from build123d import *

# Parameters (mm, degrees)
F0_W      = 60
F0_H      = 80
F2_DEPTH  = 46
F1_W      = 30
F1_H      = 10
F3_DEPTH  = 10
F4_W      = 44
F4_H      = 64
F5_DEPTH  = 30
F6_W      = 8
F6_H      = 48
F7_DEPTH  = 30
F8_W      = 22
F8_H      = 30
F8_W_2    = 8
F9_DEPTH  = 8
F10_R     = 20
F12_DEPTH = 8
F14_DEPTH = 40
F15_R     = 5
F17_DEPTH = 8
F18_R     = 5
F19_W     = 7
F19_H     = 8
F20_DEPTH = 5
F21_W     = 22
F21_H     = 30
F21_W_2   = 8
F22_DEPTH = 8
F23_SIZE2 = 29.99999
F23_SIZE  = 21.99999
F25_DEPTH = 8
F27_DEPTH = 40
F29_DEPTH = 8


# Not quite as in the source:
# - a fillet or chamfer is up to 0.001 mm smaller than in the source, because OpenCascade refuses the exact size


with BuildPart() as f2:
    # F0 (on Top) → F2 (new body)
    with BuildSketch(Plane.XY):
        Rectangle(F0_W, F0_H)
    extrude(amount=F2_DEPTH)

    # F1 (on face) → F3 (cut)
    with BuildSketch(Plane.XY):
        with Locations((-15, 30)):
            Rectangle(F1_W, F1_H)
        with Locations((15, -30)):
            Rectangle(F1_W, F1_H)
    extrude(amount=F3_DEPTH, mode=Mode.SUBTRACT)

    # F4 (on face) → F5 (cut)
    with BuildSketch(Plane.XY.offset(46)):
        Rectangle(F4_W, F4_H)
    extrude(amount=-F5_DEPTH, mode=Mode.SUBTRACT)

    # F6 (on face) → F7 (cut, through all)
    with BuildSketch(Plane.XY.offset(46)):
        with Locations((-26, 0)):
            Rectangle(F6_W, F6_H)
        with Locations((26, 0)):
            Rectangle(F6_W, F6_H)
    extrude(amount=-F7_DEPTH, mode=Mode.SUBTRACT)

    # F8 (on face) → F9 (join)
    with BuildSketch(Plane(origin=(0, -24, 0), x_dir=(-1, 0, 0), z_dir=(0, 1, 0))):
        with Locations((-41, 31)):
            Rectangle(F8_W, F8_H)
        with Locations((-26, 31)):
            Rectangle(F8_W_2, F8_H)
    extrude(amount=F9_DEPTH)

    # F10
    f10_edges = [f2.edges().sort_by_distance(p)[0] for p in [
        (52, -20, 16),
    ]]
    fillet(f10_edges, radius=F10_R)

    # F11 (on face) → F12 (join, through all)
    with BuildSketch(Plane(origin=(0, -16, 0), x_dir=(-1, 0, 0), z_dir=(0, 1, 0))):
        with BuildLine():
            ThreePointArc((-58.1533936612, 46), (-59.5344785906, 41.08453427), (-60, 36))
            ThreePointArc((-60, 36), (-51.7989898732, 16.2010101268), (-32, 8))
            Line((-32, 8), (-32, 16))
            ThreePointArc((-32, 16), (-46.1421356237, 21.8578643763), (-52, 36))
            Line((-52, 36), (-52, 46))
            Line((-52, 46), (-58.1533936612, 46))
        make_face()
        with BuildLine():
            Line((-60, 46), (-60, 36))
            ThreePointArc((-60, 36), (-59.5344785906, 41.08453427), (-58.1533936612, 46))
            Line((-58.1533936612, 46), (-60, 46))
        make_face()
        with BuildLine():
            Line((-32, 16), (-32, 8))
            ThreePointArc((-32, 8), (-30.999360817, 8.0178856906), (-30, 8.0715199125))
            Line((-30, 8.0715199125), (-30, 16))
            Line((-30, 16), (-32, 16))
        make_face()
    extrude(amount=-F12_DEPTH)

    # F13 (on face) → F14 (join, through all)
    with BuildSketch(Plane(origin=(0, -16, 0), x_dir=(-1, 0, 0), z_dir=(0, 1, 0))):
        with BuildLine():
            ThreePointArc((-58.1533936612, 46), (-59.5344785906, 41.08453427), (-60, 36))
            Line((-60, 36), (-52, 36))
            Line((-52, 36), (-52, 46))
            Line((-52, 46), (-58.1533936612, 46))
        make_face()
        with BuildLine():
            Line((-60, 46), (-60, 36))
            ThreePointArc((-60, 36), (-59.5344785906, 41.08453427), (-58.1533936612, 46))
            Line((-58.1533936612, 46), (-60, 46))
        make_face()
        with BuildLine():
            Line((-52, 36), (-60, 36))
            ThreePointArc((-60, 36), (-51.7989898732, 16.2010101268), (-32, 8))
            Line((-32, 8), (-32, 16))
            ThreePointArc((-32, 16), (-46.1421356237, 21.8578643763), (-52, 36))
        make_face()
        with BuildLine():
            Line((-32, 16), (-32, 8))
            ThreePointArc((-32, 8), (-30.999360817, 8.0178856906), (-30, 8.0715199125))
            Line((-30, 8.0715199125), (-30, 16))
            Line((-30, 16), (-32, 16))
        make_face()
    extrude(amount=F14_DEPTH)

    # F15
    f15_edges = [f2.edges().sort_by_distance(p)[0] for p in [
        (51.078784, -24, 15.506098),
    ]]
    fillet(f15_edges, radius=F15_R)

    # F16 (on face) → F17 (join)
    with BuildSketch(Plane(origin=(0, 24, 0), x_dir=(-1, 0, 0), z_dir=(0, 1, 0))):
        with BuildLine():
            ThreePointArc((-30, 8.0715199125), (-30.999360817, 8.0178856906), (-32, 8))
            Line((-32, 8), (-30, 8))
            Line((-30, 8), (-30, 8.0715199125))
        make_face()
        with BuildLine():
            Line((-30, 16), (-32, 16))
            Line((-32, 16), (-32, 8))
            ThreePointArc((-32, 8), (-30.999360817, 8.0178856906), (-30, 8.0715199125))
            Line((-30, 8.0715199125), (-30, 16))
        make_face()
        with BuildLine():
            ThreePointArc((-32, 16), (-46.1421356237, 21.8578643763), (-52, 36))
            Line((-52, 36), (-60, 36))
            ThreePointArc((-60, 36), (-51.7989898732, 16.2010101268), (-32, 8))
            Line((-32, 8), (-32, 16))
        make_face()
        with BuildLine():
            Line((-60, 46), (-60, 36))
            ThreePointArc((-60, 36), (-59.5344785906, 41.08453427), (-58.1533936612, 46))
            Line((-58.1533936612, 46), (-60, 46))
        make_face()
        with BuildLine():
            Line((-60, 36), (-52, 36))
            Line((-52, 36), (-52, 46))
            Line((-52, 46), (-58.1533936612, 46))
            ThreePointArc((-58.1533936612, 46), (-59.5344785906, 41.08453427), (-60, 36))
        make_face()
        with BuildLine():
            ThreePointArc((-30, 16.1002512579), (-30.9987444988, 16.0250785378), (-32, 16))
            Line((-32, 16), (-30, 16))
            Line((-30, 16), (-30, 16.1002512579))
        make_face()
        with BuildLine():
            ThreePointArc((-49.3205080757, 46), (-51.3185165258, 41.1763809021), (-52, 36))
            ThreePointArc((-52, 36), (-46.1421356237, 21.8578643763), (-32, 16))
            ThreePointArc((-32, 16), (-30.9987444988, 16.0250785378), (-30, 16.1002512579))
            Line((-30, 16.1002512579), (-30, 46))
            Line((-30, 46), (-49.3205080757, 46))
        make_face()
        with BuildLine():
            Line((-52, 46), (-52, 36))
            ThreePointArc((-52, 36), (-51.3185165258, 41.1763809021), (-49.3205080757, 46))
            Line((-49.3205080757, 46), (-52, 46))
        make_face()
    extrude(amount=F17_DEPTH)

    # F18
    f18_edges = [f2.edges().sort_by_distance(p)[0] for p in [
        (51.79899, 32, 16.20101),
    ]]
    fillet(f18_edges, radius=F18_R)

    # F19 (on face) → F20 (join)
    with BuildSketch(Plane.XY.offset(46)):
        with Locations((33.5, 28)):
            Rectangle(F19_W, F19_H)
        with Locations((33.5, -20)):
            Rectangle(F19_W, F19_H)
    extrude(amount=F20_DEPTH)

    # F21 (on face) → F22 (join)
    with BuildSketch(Plane.XZ.offset(-24)):
        with Locations((-41, 31)):
            Rectangle(F21_W, F21_H)
        with Locations((-26, 31)):
            Rectangle(F21_W_2, F21_H)
    extrude(amount=F22_DEPTH)

    # F23 (size 22 and 30 in the source; OpenCascade refuses exactly that, so slightly less here)
    f23_edges = [f2.edges().sort_by_distance(p)[0] for p in [
        (-52, 20, 16),
    ]]
    f23_side = f2.faces().sort_by_distance((-41, 20, 16))[0]
    chamfer(f23_edges, length=F23_SIZE, length2=F23_SIZE2, reference=f23_side)

    # F24 (on face) → F25 (join)
    with BuildSketch(Plane.XZ.offset(-16)):
        Polygon((-30, 16), (-52, 46), (-61.9205734601, 46), (-30, 2.4719452816), align=None)
    extrude(amount=-F25_DEPTH)

    # F26 (on face) → F27 (join, through all)
    with BuildSketch(Plane.XZ.offset(-16)):
        Polygon((-61.9205734601, 46), (-30, 2.4719452816), (-30, 16), (-52, 46), align=None)
    extrude(amount=F27_DEPTH)

    # F28 (on face) → F29 (join)
    with BuildSketch(Plane.XZ.offset(24)):
        Polygon((-51.9714293201, 45.961039982), (-30, 16), (-30, 45.8750016987), align=None)
        Polygon((-61.9205734601, 46), (-30, 2.4719452816), (-30, 16), (-51.9714293201, 45.961039982), align=None)
    extrude(amount=F29_DEPTH)


solid = f2.part
Could you check a few things on this model? Use its own coordinates, in mm. A direction names the side the tool comes from. Round coordinates to 2 decimals unless told otherwise and drop trailing zeros. Write each loop counter-clockwise with the first axis right and the second up, starting at its lowest first coordinate (ties: lowest second). Pieces come first, ordered by that corner, then holes. Notation, with made-up numbers: (9, 16) - (35, 16) arc R25 cw to (35, 44) - close; hole circle Ø10 at (-19, 77). An arc over 180 degrees is marked (long way). Put each result on its own line as item: value. Start each with the question number.
(1) I need wall thicknesses on probe 1 along Y at (x, z) = (38, 17); probe 2 along Y at (x, z) = (27.5, 33); probe 3 along X at (y, z) = (12.5, 37.5). Which ranges of each line are inside material? Lowest first, please.
(2) Thinking about a two-plate mould opening in Y: for faces 1 (the cylindrical face through (58, 31, 41)), 2 (the flat face through (1, 0, 16)), 3 (the flat face through (-46.184, -3.608, 24.541)), which applies, released by +Y, released by -Y, zero draft, split by the parting line, or undercut?
(3) Will these pins go through, and if not, where does the flat tip stop? pin 1 (4 mm diameter, centred on y = 22.5, z = 21.5, fed in from +X); pin 2 (10 mm diameter, centred on y = 11, z = 39, fed in from -X); pin 3 (6 mm diameter, centred on x = -40.5, z = 45.5, fed in from -Y); pin 4 (1.6 mm diameter, centred on x = 30.5, y = 25, fed in from -Z).
(4) I want a section at A-A, the plane x = 5. Please give me the cut outline in (y, z).
(5) For faces 4 (the flat face through (-26, 20, 46)), 5 (the flat face through (40, -24, 32)), 6 (the flat face through (15, -25, 5)), 7 (the flat face through (-15, 35, 5)), which set-ups out of +Z, -Z, +X, -X, +Y, -Y let a thin tool reach every point of the face, with its end or its side?
(6) I want a section at D-D, the plane z = 5.5. Please give me the cut outline in (x, y), plus the area to 3 significant figures.
(7) I want a section at B-B, the plane y = -5.5. Please give me the cut outline in (x, z), plus the area to 3 significant figures.
(8) I want a section at C-C, the plane z = 43. Please give me the cut outline in (x, y), plus the area to 3 significant figures.
Here are the results:
1. probe 1: y = -24 to -16, 24 to 32
1. probe 2: y = -40 to -16, 24 to 40
1. probe 3: x = -55.69 to -45.77, 52 to 60
2. face 1: released by +Y
2. face 2: undercut
2. face 3: zero draft
3. pin 1: stops at x = 57.05
3. pin 2: stops at x = -60.45
3. pin 3: stops at y = -32
3. pin 4: stops at z = 0
4. outline: (-40, 0) - (-35, 0) - (-35, 10) - (-25, 10) - (-25, 0) - (40, 0) - (40, 46) - (32, 46) - (32, 16) - (-32, 16) - (-32, 46) - (-40, 46) - close
5. face 4: +Z, -X, +Y, -Y
5. face 5: +Z, -Z, +X, -Y
5. face 6: -Z, +X
5. face 7: -Z, -X
6. outline: (-32.22, -32) - (-30, -32) - (-30, -40) - (30, -40) - (30, -35) - (0, -35) - (0, -25) - (30, -25) - (30, 40) - (-30, 40) - (-30, 35) - (0, 35) - (0, 25) - (-30, 25) - (-30, 24) - (-32.22, 24) - close
6. area: 4,320 mm^2
7. outline: (-61.92, 46) - (-30, 2.47) - (-30, 0) - (30, 0) - (30, 8.07) arc R28 ccw to (60, 36) - (60, 46) - (52, 46) - (52, 36) arc R20 cw to (32, 16) - (-30, 16) - (-52, 46) - close
7. area: 1,720 mm^2
8. outline: (-59.72, -32) - (-30, -32) - (-30, -40) - (30, -40) - (30, -24) - (55, -24) arc R5 ccw to (60, -19) - (60, 27) arc R5 ccw to (55, 32) - (30, 32) - (30, 40) - (-30, 40) - (-30, 24) - (-59.72, 24) - close; hole (-49.8, -24) - (-22, -24) - (-22, -32) - (22, -32) - (22, -16) - (52, -16) - (52, 24) - (22, 24) - (22, 32) - (-22, 32) - (-22, 16) - (-49.8, 16) - close
8. area: 3,010 mm^2
